from build123d import *

# Parameters (mm, degrees)
SKETCH1_R           = 1.5748
BOSS_EXTRUDE2_DEPTH = 3.175


with BuildPart() as part:
    # Sketch1 → Boss-Extrude2 (new body)
    with BuildSketch(Plane.XY):
        with BuildLine():
            Line((95.015088918, 73.039622028), (93.442430116, 67.947203051))
            Line((93.442430116, 67.947203051), (93.442430116, 65.400993562))
            Line((93.442430116, 65.400993562), (94.228759517, 62.405452988))
            Line((94.228759517, 62.405452988), (95.838862576, 58.286584697))
            Line((95.838862576, 58.286584697), (97.860852464, 54.617047494))
            Line((97.860852464, 54.617047494), (99.187742953, 52.208986977))
            Line((99.187742953, 52.208986977), (102.054609268, 48.326412287))
            Line((102.054609268, 48.326412287), (104.044945002, 44.714321512))
            Line((104.044945002, 44.714321512), (123.032849585, 15.718572297))
            add(Edge.make_bspline(
                [(123.032849585, 15.718572297), (123.714332191, 14.723172575), (125.027867192, 12.417046111), (126.13133155, 9.993338557), (127.965130812, 10.093714094)],
                knots=[0, 0, 0, 0, 0.482545384, 1, 1, 1, 1], degree=3))
            Line((127.965130812, 10.093714094), (130.045906785, 10.470125175))
            Line((130.045906785, 10.470125175), (133.787640512, 10.774684897))
            Line((133.787640512, 10.774684897), (151.974206763, 11.470821404))
            add(Edge.make_bspline(
                [(157.829388483, 14.502166506), (157.371014603, 12.448651519), (153.413195637, 11.740221824), (151.974206763, 11.470821404)],
                knots=[0, 0, 0, 0, 1, 1, 1, 1], degree=3))
            add(Edge.make_bspline(
                [(153.017246456, 28.246281812), (155.053521845, 25.097258497), (156.168563434, 23.654410632), (158.146330261, 19.312087579), (157.900569474, 15.925786313), (157.829388483, 14.502166506)],
                knots=[0, 0, 0, 0, 0.545638179, 0.593853925, 1, 1, 1, 1], degree=3))
            add(Edge.make_bspline(
                [(147.437307536, 34.637439041), (151.311718476, 32.18181338), (153.017246456, 28.246281812)],
                knots=[0, 0, 0, 1, 1, 1], degree=2))
            add(Edge.make_bspline(
                [(141.208586267, 38.180201711), (142.057807777, 37.336444115), (142.696530206, 36.831682565), (143.864835089, 34.558137065), (144.807852022, 36.057345018), (147.437307536, 34.637439041)],
                knots=[0, 0, 0, 0, 0.387994133, 0.411004513, 1, 1, 1, 1], degree=3))
            add(Edge.make_bspline(
                [(137.536109778, 43.092261061), (139.98410163, 41.245320741), (141.208586267, 38.180201711)],
                knots=[0, 0, 0, 1, 1, 1], degree=2))
            add(Edge.make_bspline(
                [(134.617377974, 47.591397428), (137.229688432, 45.916641925), (137.536109778, 43.092261061)],
                knots=[0, 0, 0, 1, 1, 1], degree=2))
            Line((134.617377974, 47.591397428), (134.513357882, 48.326412287))
            Line((134.513357882, 48.326412287), (131.916773648, 66.674098307))
            add(Edge.make_bspline(
                [(132.897509942, 76.314808247), (132.915948654, 73.197862503), (134.383448092, 69.97548856), (133.38418012, 67.42441049), (131.916773648, 66.674098307)],
                knots=[0, 0, 0, 0, 0.57532368, 1, 1, 1, 1], degree=3))
            Line((132.897509942, 76.314808247), (133.787640512, 79.197135805))
            Line((133.787640512, 79.197135805), (138.995570312, 86.101639813))
            Line((138.995570312, 86.101639813), (140.361296403, 91.450733668))
            Line((140.361296403, 91.450733668), (143.122445567, 97.027448538))
            Line((143.122445567, 97.027448538), (144.200087546, 99.203970593))
            Line((144.200087546, 99.203970593), (145.570696028, 104.572187149))
            add(Edge.make_bspline(
                [(90.14826379, 99.94311483), (116.963000062, 92.578435943), (145.570696028, 104.572187149)],
                knots=[0, 0, 0, 1, 1, 1], degree=2))
            Line((90.14826379, 99.94311483), (92.499806905, 86.943937416))
            Line((92.499806905, 86.943937416), (95.015088918, 73.039622028))
        make_face()
        with Locations((115.239537292, 84.884886181)):
            Circle(SKETCH1_R, mode=Mode.SUBTRACT)
    extrude(amount=BOSS_EXTRUDE2_DEPTH)


solid = part.part
Here's how the part is built. I have some questions about the finished solid (model axes, mm). A direction names the side the tool comes from. Coordinates: 2 decimals unless noted, no trailing zeros. Loops run counter-clockwise (first coordinate to the right, second up) from the corner with the lowest first, then second, coordinate; pieces in that order, holes last.
1. For faces 5 (the flat face through (93.83, 63.92, 1.57)), 6 (the flat face through (144.876, 101.851, 1.565)), which set-ups out of +Z, -Z, +X, -X, +Y, -Y let a thin tool reach every point of the face, with its end or its side?
2. Imagine slicing it at B-B, the plane y = 50.5. Please give me the cut outline in (x, z) (3 decimals).
3. If we mould it in two halves opening along Y, with no side actions, what happens to faces 1 (the flat face through (94.24, 70.53, 1.57)), 2 (the flat face through (128.99, 10.28, 1.57)), 3 (the flat face through (93.442, 67, 2)), 4 (the cylindrical face through (114.898, 83.348, 1.565))? For each: pulls with the +Y half, pulls with the -Y half, needs draft (parallel to the pull), parting line crosses it, or undercut.
4. I need wall thicknesses on L1, parallel to Y at x = 123, z = 1.9; L2, parallel to Y at x = 115.5, z = 2.45; L3, parallel to Y at x = 109, z = 1.85. Which ranges of each line are inside material? Lowest first, please.
5. For P1, Ø0.8, axis at y = 66, z = 2.5, coming from the -X side; P2, Ø1.9, axis at x = 115.24, y = 84.88, coming from the +Z side, each with a flat end and sliding along its axis, tell me the tip position at first contact or that it passes through.
6. Imagine slicing it at A-A, the plane y = 88. Please give me the cut outline in (x, z) (3 decimals), and give its area (3 significant figures).
Taken from the geometry:
1. face 5: +Z, -Z, -X, -Y
1. face 6: +Z, -Z, +X
2. outline: (100.45, 0) - (134.206, 0) - (134.206, 3.175) - (100.45, 3.175) - close
3. face 1: undercut
3. face 2: pulls with the -Y half
3. face 3: needs draft
3. face 4: undercut
4. L1: y = 15.77 to 98.08
4. L2: y = 27.22 to 83.33, 86.44 to 97.28
4. L3: y = 37.15 to 97.16
5. P1: stops at x = 93.44
5. P2: passes through
6. outline: (92.309, 0) - (139.48, 0) - (139.48, 3.175) - (92.309, 3.175) - close
6. area: 150 mm2
